The listing builds one solid part. Answer for the finished solid, in the listing's coordinates (mm). Give positions to 0.01 mm unless a question says otherwise; leave off trailing zeros. Order: outer loops, then holes, each group sorted by start corner. A loop starts at its lowest first (then second) coordinate and runs counter-clockwise, first axis right, second up. Notation, with made-up numbers: (-10, 59) - (7, 59) arc R25 cw to (7, 91) - close; hole circle Ø9 at (-16.5, -2). An arc over 180 degrees is marked (long way). Answer in a Markdown table with one row per item.
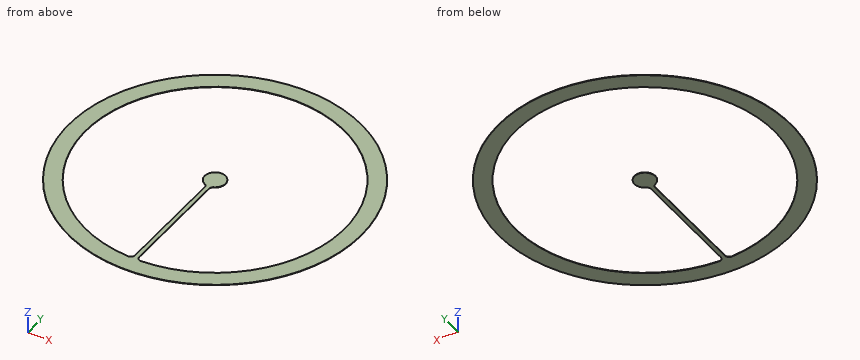
from build123d import *

# Parameters (mm, degrees)
F0_R     = 70
F1_DEPTH = 0.2
F2_R     = 2


with BuildPart() as f1:
    # F0 (on Top) → F1 (new body)
    with BuildSketch(Plane.XY):
        Circle(F0_R)
        with BuildLine():
            ThreePointArc((-1, -61.991935), (0, 62), (1, -61.991935))
            Line((1, -61.991935), (1, -4.898979))
            ThreePointArc((1, -4.898979), (0, 5), (-1, -4.898979))
            Line((-1, -4.898979), (-1, -61.991935))
        make_face(mode=Mode.SUBTRACT)
    extrude(amount=F1_DEPTH)

    # F2
    f2_edges = [f1.edges().sort_by_distance(p)[0] for p in [
        (1, -4.898979, 0.1),
        (-1, -4.898979, 0.1),
        (1, -61.991935, 0.1),
        (-1, -61.991935, 0.1),
    ]]
    fillet(f2_edges, radius=F2_R)


solid = f1.part
Item 1: Find section A-A on y = 0. Write down the section's boundary in (x, z), then the cut area to 3 significant figures.
Answer block:
| item | result |
|---|---|
| outline | (-70, 0) - (-62, 0) - (-62, 0.2) - (-70, 0.2) - close; (-5, 0) - (5, 0) - (5, 0.2) - (-5, 0.2) - close; (62, 0) - (70, 0) - (70, 0.2) - (62, 0.2) - close |
| area | 5.20 mm² |
Item 2: Find section D-D on y = 35. Write down the section's boundary in (x, z), then the cut area to 3 significant figures.
Answer block:
| item | result |
|---|---|
| outline | (-60.62, 0) - (-51.18, 0) - (-51.18, 0.2) - (-60.62, 0.2) - close; (51.18, 0) - (60.62, 0) - (60.62, 0.2) - (51.18, 0.2) - close |
| area | 3.78 mm² |
Item 3: Consider line 1 (Y direction, x = 1.5, z = 0.1); line 2 (X direction, y = -6, z = 0.15); line 3 (X direction, y = -21, z = 0.05). Determine where each line is inside the solid, lowest interval first.
Answer block:
| item | result |
|---|---|
| line 1 | -69.98 to -61.25, -5 to 4.77, 61.98 to 69.98 |
| line 2 | -69.74 to -61.71, -1.03 to 1.03, 61.71 to 69.74 |
| line 3 | -66.78 to -58.34, -1 to 1, 58.34 to 66.78 |
Item 4: Find section B-B on x = 58. Write down the section's boundary in (y, z).
Answer block:
| item | result |
|---|---|
| outline | (-39.19, 0) - (-21.91, 0) - (-21.91, 0.2) - (-39.19, 0.2) - close; (21.91, 0) - (39.19, 0) - (39.19, 0.2) - (21.91, 0.2) - close |
Item 5: Find section C-C on z = 0.1. Write down the section's boundary in (x, y).
Answer block:
| item | result |
|---|---|
| outline | circle Ø140 at (0, 0); hole (-3.1, -61.92) arc R2 ccw to (-1, -59.92) - (-1, -6.32) arc R2 ccw to (-2.14, -4.52) arc R5 cw (long way) to (2.14, -4.52) arc R2 ccw to (1, -6.32) - (1, -59.92) arc R2 ccw to (3.1, -61.92) arc R62 ccw (long way) to start |
